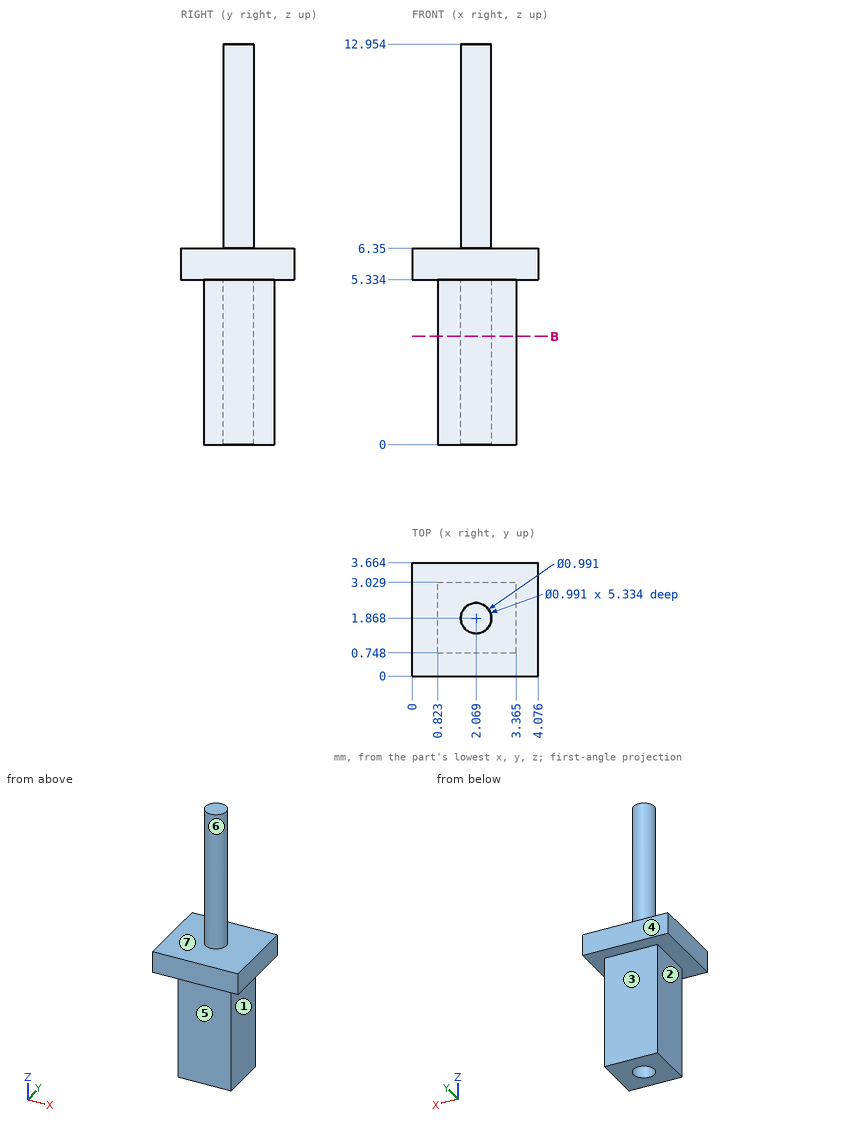
Part print with two shaded views. Sizes in mm from the minimum x, y, z corner. A direction names the side the tool comes from. Give positions to 0.01 mm unless a question says otherwise; leave off trailing zeros. Order: outer loops, then holes, each group sorted by start corner. A loop starts at its lowest first (then second) coordinate and runs counter-clockwise, first axis right, second up.
(1) Mould opens along Y. For the marked faces 4, 5, 6 and 7 say: released by +Y, released by -Y, zero draft, split by the parting line, or undercut.
(2) Drill centre lines: L1, parallel to Z at x = 3.55, y = 2; L2, parallel to Z at x = 2.45, y = 1.15; L3, parallel to Y at x = 0.95, z = 4. Where is each one in solid material? Low to high.
(3) Flat gauge pins, fed straight in: pin 1 (1.1 mm diameter, centred on x = 1, y = 1.5, fed in from +Z); pin 2 (0.7 mm diameter, centred on y = 1.5, z = 3, fed in from +X) (1 decimal); pin 3 (1.8 mm diameter, centred on y = 1.5, z = 1.5, fed in from -X). Where does each tip first touch, or does it go through?
(4) Saw through at B-B, the plane z = 3.5. Give the cut face in (x, y) (1 decimal).
(5) Tool access for the marked faces 1, 2 and 3: list every direction of +Z, -Z, +X, -X, +Y, -Y with a clear straight run to the whole face (end or side of a thin tool).
Results found:
1. face 4: released by +Y
1. face 5: released by -Y
1. face 6: split by the parting line
1. face 7: zero draft
2. L1: z = 5.33 to 6.35
2. L2: z = 0 to 6.35
2. L3: y = 0.75 to 3.03
3. pin 1: stops at z = 6.35
3. pin 2: stops at x = 3.4
3. pin 3: stops at x = 0.82
4. outline: (0.8, 0.7) - (3.4, 0.7) - (3.4, 3) - (0.8, 3) - close; hole circle Ø1 at (2.1, 1.9)
5. face 1: -Z, +X, +Y, -Y
5. face 2: -Z, -X, +Y, -Y
5. face 3: -Z, +X, -X, +Y
